Autodesk Inventor part; units mm, degrees
ref_plane "YZ Plane" through (0, 0, 0) normal (1, 0, 0) x (0, 1, 0)
ref_plane "XZ Plane" through (0, 0, 0) normal (0, 1, 0) x (-1, 0, 0)
ref_plane "XY Plane" through (0, 0, 0) normal (0, 0, 1) x (1, 0, 0)
sketch "Sketch2" plane through (0, 0, 0) normal (0, 1, 0) x (-1, 0, 0)
  line L0 (-44.45, 50.8) -> (44.45, 50.8)
  line L1 (44.45, 50.8) -> (44.45, -50.8)
  line L2 (44.45, -50.8) -> (-44.45, -50.8)
  line L3 (-44.45, -50.8) -> (-44.45, 50.8)
  point P0 (0, 0)
  dimension "d0" = 44.45
  dimension "d1" = 44.45
  dimension "d2" = 50.8
  dimension "d3" = 50.8
extrude "Extrusion1" add sketch "Sketch2" along normal blind 3.175
fillet "Fillet1" radius 12.7 4 edges at (44.45, 1.5875, 50.8) (-44.45, 1.5875, 50.8) (44.45, 1.5875, -50.8) (-44.45, 1.5875, -50.8)
sketch "Sketch3" plane through (0, 3.175, 0) normal (0, 1, 0) x (1, 0, 0)
  line L0 (-19.05, 38.1) -> (19.05, 38.1) construction
  line L1 (19.05, 38.1) -> (19.05, -38.1) construction
  line L2 (19.05, -38.1) -> (-19.05, -38.1) construction
  line L3 (-19.05, -38.1) -> (-19.05, 38.1) construction
  point P0 (0, 0)
  point P1 (0, 0)
  point P2 (-19.05, 0)
  point P3 (0, 38.1)
  dimension "d36" = 38.1
  dimension "d37" = 76.2
hole "Hole1" at (-19.05, 3.175, -38.1) at (19.05, 3.175, -38.1) at (19.05, 3.175, 38.1) at (-19.05, 3.175, 38.1) at (0, 3.175, 0) direction (0, -1, 0) diameter 6.35 end through all
sketch "Sketch4" plane through (0, 0, 0) normal (0, -1, 0) x (1, 0, 0)
  circle A0 centre (-19.05, 38.1) radius 3.175
  line L0 (44.45, -38.1) -> (44.45, 38.1)
  line L1 (-44.45, 38.1) -> (-44.45, -38.1)
  line L2 (44.45, 38.1) -> (41.275, 38.1)
  line L3 (41.275, 38.1) -> (41.275, -38.1)
  line L4 (41.275, -38.1) -> (44.45, -38.1)
  line L5 (44.45, -38.1) -> (44.45, 38.1)
  line L6 (-44.45, 38.1) -> (-41.275, 38.1)
  line L7 (-41.275, 38.1) -> (-41.275, -38.1)
  line L8 (-41.275, -38.1) -> (-44.45, -38.1)
  line L9 (-44.45, -38.1) -> (-44.45, 38.1)
  dimension "d18" = 3.175
  dimension "d19" = 3.175
  dimension "d20" = 76.2
  dimension "d21" = 76.2
extrude "Extrusion2" add sketch "Sketch4" along normal blind 120.65 contours L4 L3 L2 L0 | L6 L7 L8 L1
sketch "Sketch5" plane through (44.45, 3.175, 38.1) normal (1, 0, 0) x (0, 0, -1)
  line L0 (0, -3.175) -> (0, -123.825)
  line L1 (76.2, -3.175) -> (76.2, -123.825)
  line L2 (0, -3.175) -> (25.4, -123.825)
  line L3 (76.2, -3.175) -> (50.8, -123.825)
  line L4 (0, -3.175) -> (0, -123.825)
  line L5 (25.4, -123.825) -> (0, -123.825)
  line L6 (50.8, -123.825) -> (76.2, -123.825)
  line L7 (76.2, -123.825) -> (76.2, -3.175)
  point P0 (38.1, -3.175)
extrude "Extrusion3" cut sketch "Sketch5" against normal blind 127
sketch "Sketch6" plane through (44.45, 3.175, 38.1) normal (1, 0, 0) x (0, 0, -1)
  line L0 (25.4, -123.825) -> (50.8, -123.825)
  point P0 (38.1, -3.175)
  point P1 (38.1, -114.3)
  dimension "d28" = 9.525
hole "Hole2" at (44.45, -111.125, 0) direction (-1, 0, 0) diameter 12.7 end through all
equation "\"d4\" = metalThickness"
equation "\"d18\" = metalThickness"
equation "\"d19\" = metalThickness"
equation "\"d21\" = d20"
equation "\"metalThickness\" = 3.175"
properties part number "Caster2"
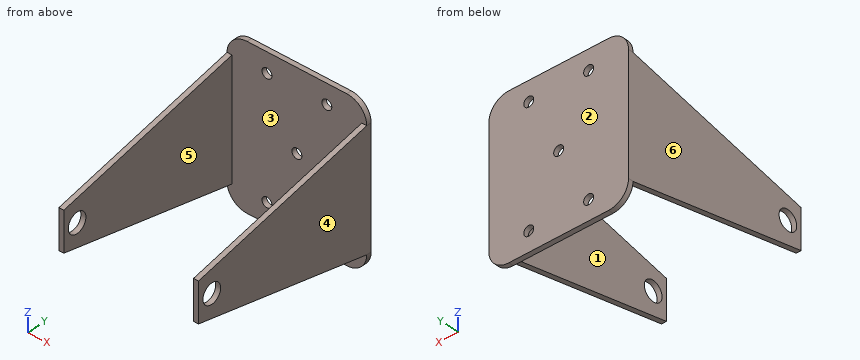
Model file for the job. Use its own axes, mm. Face numbers are marked on the shaded views. A direction names the side the tool comes from. Give positions to 0.01 mm unless a question says otherwise; leave off trailing zeros. Order: outer loops, then holes, each group sorted by start corner. A loop starts at its lowest first (then second) coordinate and runs counter-clockwise, first axis right, second up.
1) 3-axis set-ups, long thin cutter, end or side, ignore diameter. For the marked faces 5 and 6: which of +Z, -Z, +X, -X, +Y, -Y reach the whole face in a straight line?
2) Saw through at C-C, the plane x = 0. Write the cut outline in (y, z) (3 decimals), then the cut area to 3 significant figures.
3) Saw through at A-A, the plane z = 0. Write the cut outline in (x, y) (3 decimals), then the cut area to 3 significant figures.
4) Wall check: probe 1 along Z at (x, y) = (19.05, 1.35) (3 decimals); probe 2 along Y at (x, z) = (-43, 0) (3 decimals); probe 3 along X at (y, z) = (-6, 31.5) (3 decimals). Give the ranges that are in metal, low to high.
5) Mould opens along X. For the marked faces 1, 2, 3 and 4 say: +X half, -X half, draft (parallel to the pull), parting line (faces both ways), or undercut.
6) Saw through at B-B, the plane x = 19.05. Write the cut outline in (y, z) (3 decimals), then the cut area to 3 significant figures.
7) Pin check, flat tip, straight feed: pin 1 (20.5 mm diameter, centred on y = -111.125, z = 0, fed in from +X). Stop position of the tip, or through.
8) Saw through at D-D, the plane z = 18.5. Write the cut outline in (x, y) (3 decimals).
Computed:
1. face 5: +Z, -Z, -Y
1. face 6: +Z, -Z, -X, +Y, -Y
2. outline: (0, -50.8) - (3.175, -50.8) - (3.175, -3.175) - (0, -3.175) - close; (0, 3.175) - (3.175, 3.175) - (3.175, 50.8) - (0, 50.8) - close
2. area: 302 mm2
3. outline: (-44.45, -120.65) - (-41.275, -120.65) - (-41.275, -117.475) - (-44.45, -117.475) - close; (-44.45, -104.775) - (-41.275, -104.775) - (-41.275, 0) - (-3.175, 0) - (-3.175, 3.175) - (-44.45, 3.175) - close; (3.175, 0) - (41.275, 0) - (41.275, -104.775) - (44.45, -104.775) - (44.45, 3.175) - (3.175, 3.175) - close; (41.275, -120.65) - (44.45, -120.65) - (44.45, -117.475) - (41.275, -117.475) - close
3. area: 948 mm2
4. probe 1: z = -50.8 to -41.275, -34.925 to 34.925, 41.275 to 50.8
4. probe 2: y = -120.65 to -117.475, -104.775 to 3.175
4. probe 3: x = -44.45 to -41.275, 41.275 to 44.45
5. face 1: undercut
5. face 2: draft
5. face 3: undercut
5. face 4: +X half
6. outline: (0, -50.8) - (3.175, -50.8) - (3.175, -41.275) - (0, -41.275) - close; (0, -34.925) - (3.175, -34.925) - (3.175, 34.925) - (0, 34.925) - close; (0, 41.275) - (3.175, 41.275) - (3.175, 50.8) - (0, 50.8) - close
6. area: 282 mm2
7. pin 1: stops at x = 44.45
8. outline: (-44.45, -93.1) - (-41.275, -93.1) - (-41.275, 0) - (41.275, 0) - (41.275, -93.1) - (44.45, -93.1) - (44.45, 3.175) - (-44.45, 3.175) - close
